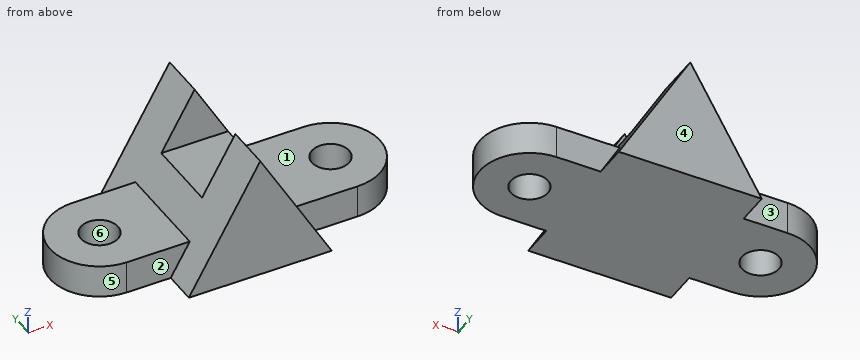
```python
from build123d import *

# Parameters (mm, degrees)
F0_R     = 7.14375
F1_DEPTH = 12.7
F3_DEPTH = 31.75
F5_DEPTH = 107.951


with BuildPart() as f1:
    # F0 (on Top) → F1 (new body)
    with BuildSketch(Plane.XY):
        with BuildLine():
            Line((0, -19.05), (88.9, -19.05))
            ThreePointArc((88.9, -19.05), (107.95, 0), (88.9, 19.05))
            Line((88.9, 19.05), (0, 19.05))
            ThreePointArc((0, 19.05), (-19.05, 0), (0, -19.05))
        make_face()
        Circle(F0_R, mode=Mode.SUBTRACT)
        with Locations((88.9, 0)):
            Circle(F0_R, mode=Mode.SUBTRACT)
    extrude(amount=F1_DEPTH)

    # F2 (on Front) → F3 (join, symmetric)
    with BuildSketch(Plane.XZ):
        Polygon((44.45, 47.625), (16.953693, 0), (44.45, 0), align=None)
        Polygon((44.45, 47.625), (44.45, 0), (71.946307, 0), align=None)
    extrude(amount=F3_DEPTH, both=True)

    # F4 (on Right) → F5 (cut, through all)
    with BuildSketch(Plane.YZ):
        Polygon((-14.2875, 25.4), (0, 25.4), (14.2875, 25.4), (14.2875, 47.625), (-14.2875, 47.625), align=None)
    extrude(amount=F5_DEPTH, mode=Mode.SUBTRACT)


solid = f1.part
```
Input: part model. Units: mm. Frame: model coordinates. Face numbers are marked on the shaded views. A direction names the side the tool comes from. Give positions to 0.01 mm unless a question says otherwise; leave off trailing zeros. Write each loop counter-clockwise with the first axis right and the second up, starting at its lowest first coordinate (ties: lowest second). Pieces come first, ordered by that corner, then holes. Notation, with made-up numbers: (-5, 2) - (20, 2) arc R17 ccw to (20, 8) - close; hole circle Ø2 at (-28.5, 36.5). An arc over 180 degrees is marked (long way). Write item = value, one per line. Start each with the question number.
1. Section query B-B, the plane z = 4.5. Output: boundary loops of the cut face in (x, y).
2. Section query D-D, the plane z = 35. Output: boundary loops of the cut face in (x, y), then the cut area to 3 significant figures.
3. Ray query, L1, parallel to Y at x = 88.9, z = 7; L2, parallel to Z at x = 67, y = 10.5; L3, parallel to Z at x = 36.5, y = -3.5. Return the intervals inside material, ascending.
4. First-contact query: pin 1 Ø2 at (y, z) = (21.5, 11) entering from -X; pin 2 Ø19 at (x, y) = (95, -0.5) entering from +Z; pin 3 Ø6 at (x, y) = (65.5, -23.5) entering from +Z. Flat tips, straight axial feed; report the tip coordinate or a pass-through.
5. Mould query, pull axis X, two halves, no side actions, for the marked faces 4, 5 and 6. Classes: released by +X, released by -X, zero draft, split by the parting line, or undercut.
6. Section query A-A, the plane y = 0. Output: boundary loops of the cut face in (x, z), then the cut area to 3 significant figures.
7. Access query for the marked faces 1, 2 and 3. Directions: +Z, -Z, +X, -X, +Y, -Y. A direction counts if a zero-diameter tool reaches every point of the face in a straight line with its end or side. Return the directions, or none.
8. Section query C-C, the plane x = -4. Output: boundary loops of the cut face in (y, z), then the cut area to 3 significant figures.
Check sheet entries:
q1.outline = (0, -19.05) - (19.55, -19.05) - (19.55, -31.75) - (69.35, -31.75) - (69.35, -19.05) - (88.9, -19.05) arc R19.05 ccw to (88.9, 19.05) - (69.35, 19.05) - (69.35, 31.75) - (19.55, 31.75) - (19.55, 19.05) - (0, 19.05) arc R19.05 ccw to start; hole circle Ø14.29 at (0, 0); hole circle Ø14.29 at (88.9, 0)
q2.outline = (37.16, -31.75) - (51.74, -31.75) - (51.74, -14.29) - (37.16, -14.29) - close; (37.16, 14.29) - (51.74, 14.29) - (51.74, 31.75) - (37.16, 31.75) - close
q2.area = 509 mm2
q3.L1 = -19.05 to -7.14, 7.14 to 19.05
q3.L2 = 0 to 12.7
q3.L3 = 0 to 25.4
q4.pin_1 = 22.73
q4.pin_2 = 12.7
q4.pin_3 = 16.36
q5.face_4 = zero draft
q5.face_5 = released by -X
q5.face_6 = undercut
q6.outline = (-19.05, 0) - (-7.14, 0) - (-7.14, 12.7) - (-19.05, 12.7) - close; (7.14, 0) - (81.76, 0) - (81.76, 12.7) - (64.61, 12.7) - (57.28, 25.4) - (31.62, 25.4) - (24.29, 12.7) - (7.14, 12.7) - close; (96.04, 0) - (107.95, 0) - (107.95, 12.7) - (96.04, 12.7) - close
q6.area = 1,670 mm2
q7.face_1 = +Z, +X, +Y, -Y
q7.face_2 = +Z, -X, -Y
q7.face_3 = +Z, -X, +Y
q8.outline = (-18.63, 0) - (-5.92, 0) - (-5.92, 12.7) - (-18.63, 12.7) - close; (5.92, 0) - (18.63, 0) - (18.63, 12.7) - (5.92, 12.7) - close
q8.area = 323 mm2
